CAD build for the part. Positions are in the model's coordinates, mm. A direction names the side the tool comes from. Round coordinates to 2 decimals unless told otherwise and drop trailing zeros. Write each loop counter-clockwise with the first axis right and the second up, starting at its lowest first coordinate (ties: lowest second). Pieces come first, ordered by that corner, then holes. Notation, with made-up numbers: (-34.5, 58.5) - (13.5, 58.5) arc R18 ccw to (13.5, 80.5) - close; hole circle Ø7 at (69.25, 85). An arc over 180 degrees is marked (long way). Use one line per item in the form item = value. Start each with the question number.
Item 1: Band-saw the part on B-B, the plane y = 4.5. List the corners of the cut face in (x, z).
Item 2: Tool access for faces 1 (the flat face through (0, 7, 0)), 2 (the flat face through (1, 9, 0)): list every direction of +Z, -Z, +X, -X, +Y, -Y with a clear straight run to the whole face (end or side of a thin tool).
Item 3: Band-saw the part on A-A, the plane z = 2.5. List the corners of the cut face in (x, y).
Item 4: Pull direction X, two halves, no side cores. Call faces 3 (the flat face through (-9, 0, 19)), 4 (the cylindrical face through (15.835, 4.437, -25.285)), 5 (the cylindrical face through (14.58, 3.45, 22.53)): +X half, -X half, draft (parallel to the pull), parting line (faces both ways), or undercut.
Item 5: Pin check, flat tips, straight feed: pin 1 (2 mm diameter, centred on y = 5.5, z = 17.5, fed in from +X); pin 2 (3 mm diameter, centred on x = -3.5, z = 7, fed in from -Y); pin 3 (1.5 mm diameter, centred on x = 11.5, y = 4.5, fed in from +Z). Stop position of each tip, or through.
Item 6: Band-saw the part on C-C, the plane x = 10.5. List the corners of the cut face in (y, z), and give its area (3 significant figures).
Item 7: Drill centre lines: L1, parallel to Y at x = -14, z = 16; L2, parallel to Z at x = 4, y = 4; L3, parallel to X at y = 4, z = 10. Where is each one in solid material? Low to high.
Autodesk Inventor part; units mm, degrees
ref_plane "YZ Plane" through (0, 0, 0) normal (1, 0, 0) x (0, 1, 0)
ref_plane "XZ Plane" through (0, 0, 0) normal (0, 1, 0) x (-1, 0, 0)
ref_plane "XY Plane" through (0, 0, 0) normal (0, 0, 1) x (1, 0, 0)
sketch "Sketch1" plane through (0, 0, 0) normal (0, 1, 0) x (-1, 0, 0)
  line L0 (72.8792, 0) -> (-46.0667, 0)
  line L1 (48.7883, 0) -> (-20.6188, 32.3651)
  line L2 (-20.6188, 32.3651) -> (-20.6188, -32.3651)
  line L3 (-20.6188, -32.3651) -> (48.7883, 0)
  circle A0 centre (-7.2188, -11.3313) radius 13.4
  circle A1 centre (-7.2188, 11.3313) radius 13.4
  circle A2 centre (17.0812, 0) radius 13.4
  circle A3 centre (0, 0) radius 20.6188
  line L4 (52.8138, 0) -> (-29.0745, 0)
  line L5 (-23.6188, -37.0741) -> (-23.6188, 37.0741)
  line L6 (-23.6188, 37.0741) -> (55.8869, 0)
  line L7 (-23.6188, -37.0741) -> (55.8869, 0)
  circle A4 centre (-7.2188, 11.3313) radius 16.4
  circle A5 centre (-7.2188, -11.3313) radius 16.4
  circle A6 centre (17.0812, 0) radius 16.4
  point P0 (-1.5557, -23.4758)
  point P1 (-20.6188, -11.3313)
  point P2 (-20.6188, 11.3313)
  point P3 (-1.5557, 23.4758)
  point P4 (22.7443, 12.1445)
  point P5 (22.7443, -12.1445)
  point P6 (-0.2879, -26.1947)
  point P7 (24.0121, -14.8634)
  point P8 (24.0121, 14.8634)
  point P9 (-0.2879, 26.1947)
  point P10 (-23.6188, 11.3313)
  point P11 (-23.6188, -11.3313)
  dimension "d9" = 50
  dimension "d10" = 26.8
  dimension "d11" = 37.7
  dimension "d12" = 26.8
  dimension "d13" = 26.8
  dimension "d14" = 3
  dimension "d15" = 3
extrude "Extrusion1" add sketch "Sketch1" along normal blind 9 contours A6 L1 A4 L6 | A6 L1 | L7 A5 L3 A6 | A6 L3 | A4 L1 | A6 L0 A2 L1 | A5 L3 | L3 A2 L0 A6 | L1 A1 L2 A4 | A5 L2 A0 L3 | A4 L2 L0 L5 | A4 L2 | L5 L0 L2 A5 | A5 L2
sketch "Sketch2" plane through (0, 9, 0) normal (0, 1, 0) x (1, 0, 0)
  line L0 (0.2879, 26.1947) -> (-24.0121, 14.8634)
  arc A0 (23.6188, 11.3313) -> (0.2879, 26.1947) centre (7.2188, 11.3313) ccw
  line L1 (23.6188, -11.3313) -> (23.6188, 11.3313)
  arc A1 (0.2879, -26.1947) -> (23.6188, -11.3313) centre (7.2188, -11.3313) ccw
  line L2 (-24.0121, -14.8634) -> (0.2879, -26.1947)
  arc A2 (-24.0121, 14.8634) -> (-24.0121, -14.8634) centre (-17.0812, 0) ccw
  arc A3 (20.6188, 11.3313) -> (1.5557, 23.4758) centre (7.2188, 11.3313) ccw
  line L3 (-22.7443, 12.1445) -> (1.5557, 23.4758)
  arc A4 (-22.7443, 12.1445) -> (-22.7443, -12.1445) centre (-17.0812, 0) ccw
  line L4 (1.5557, -23.4758) -> (-22.7443, -12.1445)
  arc A5 (1.5557, -23.4758) -> (20.6188, -11.3313) centre (7.2188, -11.3313) ccw
  line L5 (20.6188, 11.3313) -> (20.6188, -11.3313)
extrude "Extrusion2" add sketch "Sketch2" against normal blind 2 contours L5 A5 L4 A4 L3 A3
properties part number "Tri_Box"
Determined:
q1.outline = (-24.01, -14.86) - (0.29, -26.19) arc R16.4 ccw to (23.62, -11.33) - (23.62, 11.33) arc R16.4 ccw to (0.29, 26.19) - (-24.01, 14.86) arc R16.4 ccw to start; hole (-22.74, -12.14) - (1.56, -23.48) arc R13.4 ccw to (20.62, -11.33) - (20.62, 11.33) arc R13.4 ccw to (1.56, 23.48) - (-22.74, 12.14) arc R13.4 ccw to start
q2.face_1 = -Y
q2.face_2 = +Z, -Z, +X, -X, +Y
q3.outline = (-33.29, 0) - (-30.25, 0) - (-30.25, 7) - (20.62, 7) - (20.62, 0) - (23.62, 0) - (23.62, 9) - (-33.29, 9) - close
q4.face_3 = draft
q4.face_4 = parting line
q4.face_5 = undercut
q5.pin_1 = 22.78
q5.pin_2 = 7
q5.pin_3 = 27.35
q6.outline = (0, -27.4) - (9, -27.4) - (9, 27.4) - (0, 27.4) - (0, 24.32) - (7, 24.32) - (7, -24.32) - (0, -24.32) - close
q6.area = 153 mm²
q7.L1 = 7 to 9
q7.L2 = -27.41 to -24.34, 24.34 to 27.41
q7.L3 = -30.08 to -26, 20.62 to 23.62
